from build123d import *

# Parameters (mm, degrees)
ESQUISSE1_R                  = 49
BASE_EXTRUSION_DEPTH         = 30
ESQUISSE20_R                 = 3
ENL_V_MAT_EXTRU_4_DEPTH      = 12
ESQUISSE3_R                  = 10
BOSS_EXTRU_1_DEPTH           = 61
ESQUISSE11_R                 = 3
ENL_V_MAT_EXTRU_3_DEPTH      = 31.0000001
R_P_TITION_CIRCULAIRE1_COUNT = 6
R_P_TITION_CIRCULAIRE3_COUNT = 2
R_P_TITION_CIRCULAIRE3_ANGLE = 135
R_P_TITION_CIRCULAIRE4_COUNT = 3


with BuildPart() as part:
    # Esquisse1 → Base-Extrusion (new body)
    with BuildSketch(Plane.XY):
        Circle(ESQUISSE1_R)
    extrude(amount=BASE_EXTRUSION_DEPTH)

    # Esquisse2 → Boss.-Révol.1 (revolve)
    with BuildSketch(Plane(origin=(0, 0, 0), x_dir=(0, 0, -1), z_dir=(1, 0, 0))):
        Polygon((-30, 0), (-30, 17.5), (-34, 13.5), (-34, 0), align=None)
    revolve(axis=Axis((0, 0, 38.858858859), (0, 0, -1)))

    # Esquisse20 → Enlèv. mat.-Extru.4 (cut)
    with BuildSketch(Plane(origin=(-49, 0, 15), x_dir=(0, 1, 0), z_dir=(-1, 0, 0))):
        with Locations((0, -3)):
            Circle(ESQUISSE20_R)
    extrude(amount=-ENL_V_MAT_EXTRU_4_DEPTH, mode=Mode.SUBTRACT)

    # Esquisse3 → Boss.-Extru.1 (add)
    with BuildSketch(Plane.XY.offset(34)):
        Circle(ESQUISSE3_R)
    extrude(amount=BOSS_EXTRU_1_DEPTH)

    # Esquisse11 → Enlèv. mat.-Extru.3 (cut, through all)
    with BuildSketch(Plane.XY.offset(30)):
        with Locations((-22, -38.105117767)):
            Circle(ESQUISSE11_R)
    extrude(amount=-ENL_V_MAT_EXTRU_3_DEPTH, mode=Mode.SUBTRACT)

    # Esquisse12 → Perçage2 (revolve, cut)
    with BuildSketch(Plane(origin=(0, -44, 30), x_dir=(0, -1, 0), z_dir=(1, 0, 0))):
        Polygon((0, 0), (0, 26.47511282), (2.455, 25), (2.455, 0), align=None)
    per_age2 = revolve(axis=Axis((0, -44, 34.244199587), (0, 0, -1)), mode=Mode.SUBTRACT)

    # Répétition circulaire1: Perçage2 ×6 about axis
    r_p_tition_circulaire1_axis = Axis((0, 0, 0), (0, 0, 1))
    for i in range(1, R_P_TITION_CIRCULAIRE1_COUNT):
        add(per_age2.rotate(r_p_tition_circulaire1_axis, i * 360 / R_P_TITION_CIRCULAIRE1_COUNT), mode=Mode.SUBTRACT)

    # Esquisse16 → Perçage4 (revolve, cut)
    with BuildSketch(Plane(origin=(-21.242014496, 21.184353192, 0), x_dir=(0, 1, 0), z_dir=(1, 0, 0))):
        Polygon((0, 0), (0, 21.802581857), (3, 20), (3, 0), align=None)
    per_age4 = revolve(axis=Axis((-21.242014496, 21.184353192, -6.35), (0, 0, 1)), mode=Mode.SUBTRACT)

    # Répétition circulaire3: Perçage4 ×2 about axis
    r_p_tition_circulaire3_axis = Axis((0, 0, 0), (0, 0, -1))
    for i in range(1, R_P_TITION_CIRCULAIRE3_COUNT):
        add(per_age4.rotate(r_p_tition_circulaire3_axis, i * R_P_TITION_CIRCULAIRE3_ANGLE / (R_P_TITION_CIRCULAIRE3_COUNT - 1)), mode=Mode.SUBTRACT)

    # Esquisse18 → Perçage5 (revolve, cut)
    with BuildSketch(Plane(origin=(-30, -0.050785262, 0), x_dir=(0, 1, 0), z_dir=(1, 0, 0))):
        Polygon((0, 0), (0, 21.502151548), (2.5, 20), (2.5, 0), align=None)
    per_age5 = revolve(axis=Axis((-30, -0.050785262, -6.35), (0, 0, 1)), mode=Mode.SUBTRACT)

    # Répétition circulaire4: Perçage5 ×3 about axis
    r_p_tition_circulaire4_axis = Axis((0, 0, 0), (0, 0, 1))
    for i in range(1, R_P_TITION_CIRCULAIRE4_COUNT):
        add(per_age5.rotate(r_p_tition_circulaire4_axis, i * 360 / R_P_TITION_CIRCULAIRE4_COUNT), mode=Mode.SUBTRACT)

    # Groove Sketch → Retaining Ring Groove (revolve, cut)
    with BuildSketch(Plane(origin=(2.765923972, 3.631297113, 10.621036492), x_dir=(-0.506744947, -0.665289965, 0.548268931), z_dir=(0.795513937, -0.60593529, 0))):
        with BuildLine():
            Line((53.007122247, -54.964355603), (53.316554018, -54.761496098))
            Line((53.316554018, -54.761496098), (52.603804408, -53.674303387))
            Line((52.603804408, -53.674303387), (52.294372636, -53.877162891))
            ThreePointArc((52.294372636, -53.877162891), (52.238372455, -53.959405037), (52.256928326, -54.057157123))
            Line((52.256928326, -54.057157123), (52.827128014, -54.926911293))
            ThreePointArc((52.827128014, -54.926911293), (52.90937016, -54.982911474), (53.007122247, -54.964355603))
        make_face()
    revolve(axis=Axis((0, 0, 52.503783955), (0, 0, -1)), mode=Mode.SUBTRACT)


solid = part.part
CAD build for the part. Positions are in the model's coordinates, mm. A direction names the side the tool comes from. Give positions to 0.01 mm unless a question says otherwise; leave off trailing zeros. Loops run counter-clockwise (first coordinate to the right, second up) from the corner with the lowest first, then second, coordinate; pieces in that order, holes last. Notation, with made-up numbers: M -11,-37.5 L 2,-37.5 A26 ccw 2,-10.5 Z; hole C -13,-33.75 d3. An arc over 180 degrees is marked long. Answer in a Markdown table with one row per item. Add a question column.
Item 1: Drop flat-ended pins along their axis: P1, Ø5.5, axis at x = 30, y = 0.04, coming from the +Z side; P2, Ø12, axis at y = 19.5, z = 25, coming from the +X side; P3, Ø16, axis at x = -1.5, y = 3, coming from the -Z side; P4, Ø1.5, axis at x = -4.5, z = 57, coming from the +Y side. Give the stop position or say it passes through.
Item 2: Band-saw the part on A-A on z = 25.5. Give the cut face in (x, y) (1 decimal).
Item 3: Mould opens along X. For faces 1 (the face through (30.32, 0.45, 21.49)), 2 (the face through (-1, -21, 30)), 3 (the face through (-37, 0, 18)) say: +X half, -X half, draft (parallel to the pull), parting line (faces both ways), or undercut.
Item 4: Band-saw the part on B-B on z = 73.5. Give the cut face in (x, y).
Item 5: Band-saw the part on C-C on y = 36.5. Give the cut face in (x, z), then the cut area to 3 significant figures.
Item 6: Probe probe 1 along Y at (x, z) = (-1.5, 13); probe 2 along X at (y, z) = (43.5, 24.5); probe 3 along Z at (x, y) = (0, -22). List the from-to ranges inside material, lowest first.
Item 7: Tool access for faces 4 (the face through (-7.76, -5.48, 85.01)), 5 (the face through (0.108, 41.547, 17.675)), 6 (the face through (0, 0, 95)): list every direction of +Z, -Z, +X, -X, +Y, -Y with a clear straight run to the whole face (end or side of a thin tool).
Reply:
| question | item | result |
|---|---|---|
| 1 | P1 | stops at z = 30 |
| 1 | P2 | stops at x = 47.1 |
| 1 | P3 | stops at z = 0 |
| 1 | P4 | stops at y = 9.27 |
| 2 | outline | C 0,0 d98; hole C -38.1,-22 d4.9; hole C -38.1,22 d4.9; hole C -22,-38.1 d6; hole C 0,-44 d4.9; hole C 0,44 d4.9; hole C 38.1,-22 d4.9; hole C 38.1,22 d4.9 |
| 3 | face 1 | undercut |
| 3 | face 2 | draft |
| 3 | face 3 | -X half |
| 4 | outline | C 0,0 d20 |
| 5 | outline | M -32.69,0 L 32.69,0 L 32.69,30 L -32.69,30 Z |
| 5 | area | 1,960 mm^2 |
| 6 | probe 1 | y = -48.98 to -45.94, -42.06 to 42.06, 45.94 to 48.98 |
| 6 | probe 2 | x = -22.56 to -2.4, 2.4 to 22.56 |
| 6 | probe 3 | z = 0 to 30 |
| 7 | face 4 | none |
| 7 | face 5 | +Z |
| 7 | face 6 | +Z, +X, -X, +Y, -Y |
